```python
from build123d import *

# Parameters (mm, degrees)
CROQUIS2_W              = 66.675
CROQUIS2_H              = 66.675
SALIENTE_EXTRUIR2_DEPTH = 88.9
CORTAR_EXTRUIR1_DEPTH   = 117.01790608
CROQUIS4_R              = 25.4
CORTAR_EXTRUIR2_DEPTH   = 19.05
CORTAR_EXTRUIR3_DEPTH   = 31.75
CROQUIS6_OUTSIDE_W      = 94.593
CROQUIS6_OUTSIDE_H      = 94.593
CROQUIS6_OUTSIDE_R      = 33.3375
CORTAR_EXTRUIR5_DEPTH   = 101.627967348
CORTAR_EXTRUIR6_DEPTH   = 50.8
CROQUIS9_R              = 3.175
CORTAR_EXTRUIR7_DEPTH   = 60.325


with BuildPart() as part:
    # Croquis2 → Saliente-Extruir2 (new body)
    with BuildSketch(Plane.XY):
        Rectangle(CROQUIS2_W, CROQUIS2_H)
    extrude(amount=SALIENTE_EXTRUIR2_DEPTH)

    # Croquis3 → Cortar-Extruir1 (cut, through all)
    with BuildSketch(Plane(origin=(33.3375, 0, 0), x_dir=(0, 0, -1), z_dir=(1, 0, 0))):
        Polygon((-88.9, 0), (-88.9, 33.3375), (-31.157756203, 33.3375), align=None)
    extrude(amount=-CORTAR_EXTRUIR1_DEPTH, mode=Mode.SUBTRACT)

    # Croquis4 → Cortar-Extruir2 (cut)
    with BuildSketch(Plane.XY.offset(88.9)):
        Circle(CROQUIS4_R)
    extrude(amount=-CORTAR_EXTRUIR2_DEPTH, mode=Mode.SUBTRACT)

    # Croquis5 → Cortar-Extruir3 (cut)
    with BuildSketch(Plane.XY.offset(69.85)):
        with BuildLine():
            Line((-9.525, -7.9248), (-9.525, 33.3375))
            Line((-9.525, 33.3375), (9.525, 33.3375))
            Line((9.525, 33.3375), (9.525, -7.9248))
            ThreePointArc((9.525, -7.9248), (0, -17.4498), (-9.525, -7.9248))
        make_face()
    extrude(amount=-CORTAR_EXTRUIR3_DEPTH, mode=Mode.SUBTRACT)

    # Croquis6 outside → Cortar-Extruir5 (cut, through all)
    with BuildSketch(Plane.XY.offset(88.9)):
        with Locations((0.0005, 0.0005)):
            Rectangle(CROQUIS6_OUTSIDE_W, CROQUIS6_OUTSIDE_H)
        Circle(CROQUIS6_OUTSIDE_R, mode=Mode.SUBTRACT)
    extrude(amount=-CORTAR_EXTRUIR5_DEPTH, mode=Mode.SUBTRACT)

    # Croquis8 → Cortar-Extruir6 (cut)
    with BuildSketch(Plane.XY.offset(88.9)):
        with BuildLine():
            Line((-30.1752, 14.172022128), (-30.1752, -14.172022128))
            ThreePointArc((-30.1752, -14.172022128), (-33.3375, 0), (-30.1752, 14.172022128))
        make_face()
        with BuildLine():
            Line((30.1498, 14.225978568), (30.1498, -14.225978568))
            ThreePointArc((30.1498, -14.225978568), (33.3375, 0), (30.1498, 14.225978568))
        make_face()
    extrude(amount=-CORTAR_EXTRUIR6_DEPTH, mode=Mode.SUBTRACT)

    # Croquis9 → Cortar-Extruir7 (cut)
    with BuildSketch(Plane(origin=(30.1498, 0, 0), x_dir=(0, 0, -1), z_dir=(1, 0, 0))):
        with Locations((-57.15, 7.9248)):
            Circle(CROQUIS9_R)
    extrude(amount=-CORTAR_EXTRUIR7_DEPTH, mode=Mode.SUBTRACT)


solid = part.part
```
Work out the finished part from the listing and answer in its coordinate system (mm). A direction names the side the tool comes from. Round coordinates to 2 decimals unless told otherwise and drop trailing zeros. Write each loop counter-clockwise with the first axis right and the second up, starting at its lowest first coordinate (ties: lowest second). Pieces come first, ordered by that corner, then holes.
1) A cutting plane is placed at D-D on y = 6. Determine the outline of the cut face in (x, z) (3 decimals), and give its area (3 significant figures).
2) Determine the mould class of faces 1 (the face through (19.982, 6.709, 54.217)), 2 (the face through (30.15, -3, 64)), 3 (the face through (-7.227, -32.545, 35.195)) for opening direction Y: pulls with the +Y half, pulls with the -Y half, needs draft (parallel to the pull), parting line crosses it, or undercut.
3) A cutting plane is placed at B-B on z = 57.15. Give the number of separate pieces and of enclosed holes in the cut face, and give its area (3 significant figures).
4) Flat-ended cylindrical pins translate along their axes: P1, Ø9.5, axis at y = 13, z = 62, coming from the -X side; P2, Ø8, axis at x = 24.5, z = 72.5, coming from the +Y side; P3, Ø8.5, axis at y = 7.92, z = 57.15, coming from the +X side. Find the tip coordinate at first contact, or state that the pin passes through.
5) A cutting plane is placed at A-A on x = 0. Determine the outline of the cut face in (y, z), and give its area (3 significant figures).
6) Consider probe 1 along X at (y, z) = (-6.5, 44.5) (3 decimals); probe 2 along X at (y, z) = (0, 78); probe 3 along Y at (x, z) = (0, 25.5). Determine where each line is inside the solid, lowest interval first.
7) Which of the six approach directions +Z, -Z, +X, -X, +Y, -Y give full straight-line access (tool end or side, diameter ignored) to faces 4 (the face through (-0.72, -25.39, 79.51)), 5 (the face through (9.525, 7, 51)), 6 (the face through (31, 0, 38.1)), 7 (the face through (-30.175, -3, 64))?
Entries:
1. outline: (-32.793, 0) - (32.793, 0) - (32.793, 38.1) - (30.15, 38.1) - (30.15, 54.625) - (9.525, 54.625) - (9.525, 38.1) - (-9.525, 38.1) - (-9.525, 54.625) - (-30.175, 54.625) - (-30.175, 38.1) - (-32.793, 38.1) - close; (-30.175, 59.675) - (-9.525, 59.675) - (-9.525, 69.85) - (-24.681, 69.85) - (-24.681, 78.508) - (-30.175, 78.508) - close; (9.525, 59.675) - (30.15, 59.675) - (30.15, 78.508) - (24.681, 78.508) - (24.681, 69.85) - (9.525, 69.85) - close
1. area: 3,700 mm2
2. face 1: undercut
2. face 2: needs draft
2. face 3: parting line crosses it
3. separate pieces: 3
3. enclosed holes: 0
3. area: 1,880 mm2
4. P1: stops at x = -30.18
4. P2: stops at y = 11.78
4. P3: stops at x = 30.15
5. outline: (-33.34, 0) - (33.34, 0) - (33.34, 31.16) - (29.33, 38.1) - (-17.45, 38.1) - (-17.45, 69.85) - (-25.4, 69.85) - (-25.4, 88.9) - (-33.34, 88.9) - close
5. area: 3,180 mm2
6. probe 1: x = -30.175 to -9.525, 9.525 to 30.15
6. probe 2: x = -30.18 to -25.4, 25.4 to 30.15
6. probe 3: y = -33.34 to 33.34
7. face 4: +Z
7. face 5: +Z, +Y
7. face 6: +Z, +X, +Y, -Y
7. face 7: +Z, -X, +Y, -Y
